```python
from build123d import *

# Parameters (mm, degrees)
BOSS_EXTRUDE1_DEPTH = 0.79375
SKETCH2_R           = 3.175
BOSS_EXTRUDE2_DEPTH = 3.175
SKETCH3_R           = 1.7859375
CUT_EXTRUDE1_DEPTH  = 6.35


with BuildPart() as part:
    # Sketch1 → Boss-Extrude1 (new body)
    with BuildSketch(Plane.XY):
        with BuildLine():
            ThreePointArc((-4.10493597, 2.24506403), (-9.525, 0), (-4.10493597, -2.24506403))
            add(Edge.make_bspline(
                [(-4.10493597, -2.24506403), (0, 0.65756403), (4.10493597, -2.24506403)],
                knots=[0, 0, 0, 1, 1, 1], degree=2))
            ThreePointArc((4.10493597, -2.24506403), (9.525, 0), (4.10493597, 2.24506403))
            add(Edge.make_bspline(
                [(-4.10493597, 2.24506403), (0, -0.65756403), (4.10493597, 2.24506403)],
                knots=[0, 0, 0, 1, 1, 1], degree=2))
        make_face()
    boss_extrude1 = extrude(amount=BOSS_EXTRUDE1_DEPTH)

    # Sketch2 → Boss-Extrude2 (add)
    with BuildSketch(Plane.XY.offset(0.79375)):
        with Locations(Location((-6.35, 0, 0), (0, 0, 315))):
            Circle(SKETCH2_R)
        with Locations(Location((6.35, 0, 0), (0, 0, 135))):
            Circle(SKETCH2_R)
    extrude(amount=BOSS_EXTRUDE2_DEPTH)

    # Mirror1: Boss-Extrude1 across plane
    add(boss_extrude1.mirror(Plane.XY.offset(2.38125)))

    # Sketch3 → Cut-Extrude1 (cut)
    with BuildSketch(Plane(origin=(0, 0, 0), x_dir=(-1, 0, 0), z_dir=(0, 0, -1))):
        with Locations((-6.35, 0)):
            Circle(SKETCH3_R)
        with Locations((6.35, 0)):
            Circle(SKETCH3_R)
    extrude(amount=-CUT_EXTRUDE1_DEPTH, mode=Mode.SUBTRACT)


solid = part.part
```
The model under review builds one solid part; all positions refer to its coordinate system, in mm. Round coordinates to 2 decimals unless told otherwise and drop trailing zeros. Order: outer loops, then holes, each group sorted by start corner. A loop starts at its lowest first (then second) coordinate and runs counter-clockwise, first axis right, second up. Notation, with made-up numbers: M 25,-19.75 L 65,-19.75 A22 cw 65,-0.75 Z; hole C -8,-16.5 d5. An arc over 180 degrees is marked long. Use a Markdown table: item, result.
1) Consider section C-C (z = 2.6). Write out the cut boundary in (x, y) (3 decimals).
Report:
| item | result |
|---|---|
| outline | C -6.35,0 d6.35; C 6.35,0 d6.35; hole C -6.35,0 d3.572; hole C 6.35,0 d3.572 |
2) Consider section D-D (z = 0.3). Give the number of separate pieces and of enclosed holes in the cut face, then the cut area to 3 significant figures.
Report:
| item | result |
|---|---|
| separate pieces | 1 |
| enclosed holes | 2 |
| area | 58.5 mm^2 |
3) Insertion check: pin 1 (2 mm diameter, centred on x = 6.35, y = 0, fed in from +Z). The pin has a flat end and moves straight along its axis. Give the tip position at first contact, or say it passes through.
Report:
| item | result |
|---|---|
| pin 1 | through |
4) Wall thickness on line 1 along Z through (x, y) = (-2, 1); line 2 along Y through (x, z) = (-6.35, 1.1) (3 decimals); line 3 along X through (y, z) = (-1.5, 0.6): over which ranges is each line inside the solid? List them lowest first. Write a range as [from, to].
Report:
| item | result |
|---|---|
| line 1 | [0, 0.79], [3.97, 4.76] |
| line 2 | [-3.175, -1.786], [1.786, 3.175] |
| line 3 | [-9.15, -7.32], [-5.38, -2.86], [2.86, 5.38], [7.32, 9.15] |
5) Consider section A-A (x = 6.35). Write out the cut boundary in (y, z) (1 decimal), then the cut area to 3 significant figures.
Report:
| item | result |
|---|---|
| outline | M -3.2,0 L -1.8,0 L -1.8,4.8 L -3.2,4.8 Z; M 1.8,0 L 3.2,0 L 3.2,4.8 L 1.8,4.8 Z |
| area | 13.2 mm^2 |
6) Draft analysis for pull direction X (two halves, no side actions). For faces 1 (the face through (-4.566, 0.079, 2.348)), 2 (the face through (0, 0, 0)), 3 (the face through (0, 0, 0.794)), state which applies: released by +X, released by -X, zero draft, split by the parting line, or undercut.
Report:
| item | result |
|---|---|
| face 1 | undercut |
| face 2 | zero draft |
| face 3 | undercut |
7) Consider section B-B (y = 0). Write out the cut boundary in (x, z) (1 decimal).
Report:
| item | result |
|---|---|
| outline | M -9.5,0 L -8.1,0 L -8.1,4.8 L -9.5,4.8 Z; M -4.6,0 L 4.6,0 L 4.6,4.8 L -4.6,4.8 Z; M 8.1,0 L 9.5,0 L 9.5,4.8 L 8.1,4.8 Z; hole M -3.2,0.8 L 3.2,0.8 L 3.2,4 L -3.2,4 Z |
